```python
from build123d import *

# Parameters (mm, degrees)
F0_W     = 25.4
F0_H     = 50.8
F0_R     = 6.35
F1_DEPTH = 12.7
F3_D     = 12.7
F4_R     = 5.08


with BuildPart() as f1:
    # F0 (on Top) → F1 (new body, symmetric)
    with BuildSketch(Plane.XY):
        Rectangle(F0_W, F0_H)
        with Locations((0, 12.7)):
            Circle(F0_R, mode=Mode.SUBTRACT)
    extrude(amount=F1_DEPTH, both=True)

    # F3 (through all)
    with Locations(Plane(origin=(-12.7, 0, 0), x_dir=(0, -1, 0), z_dir=(-1, 0, 0))):
        with Locations((12.7, 0)):
            Hole(F3_D / 2)

    # F4
    f4_edges = [f1.edges().sort_by_distance(p)[0] for p in [
        (0, -25.4, -12.7),
        (12.7, -25.4, 0),
        (0, -25.4, 12.7),
        (-12.7, -25.4, 0),
        (12.7, 25.4, 0),
        (0, 25.4, -12.7),
        (-12.7, 25.4, 0),
        (0, 25.4, 12.7),
        (-12.7, 0, -12.7),
        (12.7, 0, -12.7),
        (12.7, 0, 12.7),
        (-12.7, 0, 12.7),
    ]]
    fillet(f4_edges, radius=F4_R)


solid = f1.part
```
Could you check a few things on this model? Use its own coordinates, in mm. Coordinates: 2 decimals unless noted, no trailing zeros. Loops run counter-clockwise (first coordinate to the right, second up) from the corner with the lowest first, then second, coordinate; pieces in that order, holes last. Notation, with made-up numbers: M 23,-2 L 50,-2 A10 ccw 50,2 Z; hole C 8,-31 d1. An arc over 180 degrees is marked long. Put each result on its own line as item: value. Start each with the question number.
(1) Suppose I cut it at D-D on y = -3.5. Please give me the cut outline in (x, z), then the cut area to 3 significant figures.
(2) Suppose I cut it at C-C on y = 12.7. Please give me the cut outline in (x, z).
(3) Suppose I cut it at B-B on z = 0. Please give me the cut outline in (x, y).
(4) I need wall thicknesses on line 1 (Y direction, x = 0, z = -3.25); line 2 (Y direction, x = 2.25, z = -3); line 3 (Z direction, x = -7, y = -12.5). Which ranges of each line are inside material? Lowest first, please. Write a range as from..to.
(5) Thinking about a two-plate mould opening in Y: for faces 1 (the face through (0.107, -23.951, -11.172)), 2 (the face through (-11.251, 0.284, 11.172)), 3 (the face through (3.414, 18.054, -0.178)), 4 (the face through (0.178, -6.643, 1.907)), which applies, pulls with the +Y half, pulls with the -Y half, needs draft (parallel to the pull), parting line crosses it, or undercut?
(6) Will this pin go through, and if not, where does the flat tip stop? P1, Ø2, axis at x = -10, y = -3.5, coming from the -Z side.
(7) Suppose I cut it at A-A on x = 0. Please give me the cut outline in (y, z).
Solutions:
1. outline: M -12.7,-7.62 A5.08 ccw -7.62,-12.7 L 7.62,-12.7 A5.08 ccw 12.7,-7.62 L 12.7,7.62 A5.08 ccw 7.62,12.7 L -7.62,12.7 A5.08 ccw -12.7,7.62 Z
1. area: 623 mm2
2. outline: M -12.7,-7.62 A5.08 ccw -7.62,-12.7 L -6.35,-12.7 L -6.35,12.7 L -7.62,12.7 A5.08 ccw -12.7,7.62 Z; M 6.35,-12.7 L 7.62,-12.7 A5.08 ccw 12.7,-7.62 L 12.7,7.62 A5.08 ccw 7.62,12.7 L 6.35,12.7 Z
3. outline: M -12.7,-20.32 A5.08 ccw -7.62,-25.4 L 7.62,-25.4 A5.08 ccw 12.7,-20.32 L 12.7,-19.05 L -12.7,-19.05 Z; M -12.7,-6.35 L 12.7,-6.35 L 12.7,20.32 A5.08 ccw 7.62,25.4 L -7.62,25.4 A5.08 ccw -12.7,20.32 Z; hole C 0,12.7 d12.7
4. line 1: y = -25.4..-18.16, -7.24..6.35, 19.05..25.4
4. line 2: y = -25.4..-18.3, -7.1..6.76, 18.64..25.4
4. line 3: z = -12.7..-6.35, 6.35..12.7
5. face 1: pulls with the -Y half
5. face 2: needs draft
5. face 3: undercut
5. face 4: undercut
6. P1: stops at z = -12.51
7. outline: M -25.4,-7.62 A5.08 ccw -20.32,-12.7 L 6.35,-12.7 L 6.35,12.7 L -20.32,12.7 A5.08 ccw -25.4,7.62 Z; M 19.05,-12.7 L 20.32,-12.7 A5.08 ccw 25.4,-7.62 L 25.4,7.62 A5.08 ccw 20.32,12.7 L 19.05,12.7 Z; hole C -12.7,0 d12.7
